```python
from build123d import *

# Parameters (mm, degrees)
BOSS_EXTRUDE1_DEPTH = 20
FILLET2_R           = 2.5
SKETCH2_R           = 2.5
CUT_EXTRUDE1_DEPTH  = 10
SKETCH3_R           = 2.5
CUT_EXTRUDE2_DEPTH  = 10


with BuildPart() as part:
    # Sketch1 → Boss-Extrude1 (new body)
    with BuildSketch(Plane.XY):
        Polygon((0, 0), (20, 0), (20, 18.325792173), (42, 18.325792173), (42, 1.536318489), (62, 1.536318489), (62, 5.536318489), (46, 5.536318489), (46, 22.325792173), (16, 22.325792173), (16, 4), (0, 4), align=None)
    extrude(amount=BOSS_EXTRUDE1_DEPTH)

    # Fillet2
    fillet2_edges = [part.edges().sort_by_distance(p)[0] for p in [
        (16, 4, 10),
        (16, 22.325792173, 10),
        (46, 22.325792173, 10),
        (46, 5.536318489, 10),
    ]]
    fillet(fillet2_edges, radius=FILLET2_R)

    # Sketch2 → Cut-Extrude1 (cut)
    with BuildSketch(Plane(origin=(0, 4, 0), x_dir=(1, 0, 0), z_dir=(0, 1, 0))):
        with Locations((7, -10)):
            Circle(SKETCH2_R)
    extrude(amount=-CUT_EXTRUDE1_DEPTH, mode=Mode.SUBTRACT)

    # Sketch3 → Cut-Extrude2 (cut)
    with BuildSketch(Plane(origin=(0, 5.536318489, 0), x_dir=(1, 0, 0), z_dir=(0, 1, 0))):
        with Locations((55, -10)):
            Circle(SKETCH3_R)
    extrude(amount=-CUT_EXTRUDE2_DEPTH, mode=Mode.SUBTRACT)


solid = part.part
```
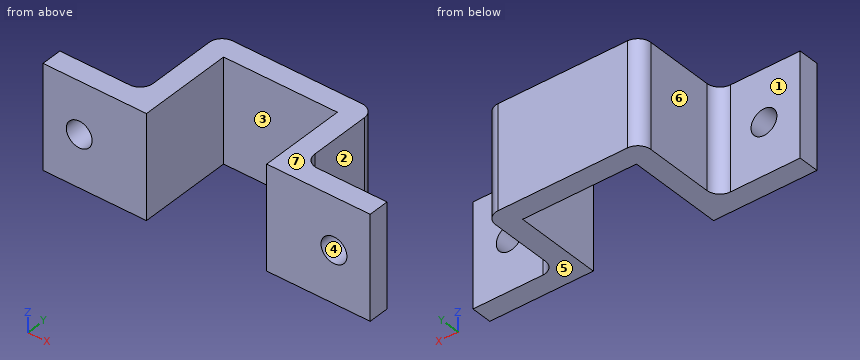
Could you check a few things on this model? Use its own coordinates, in mm. Face numbers are marked on the shaded views. A direction names the side the tool comes from. Coordinates: 2 decimals unless noted, no trailing zeros. Loops run counter-clockwise (first coordinate to the right, second up) from the corner with the lowest first, then second, coordinate; pieces in that order, holes last.
1) Which directions (+Z, -Z, +X, -X, +Y, -Y) give clear straight access to the entire face, cutting with the end or side of a thin tool? Please do the marked faces 1, 2 and 3.
Reported:
face 1: +Z, -Z, -X, +Y
face 2: +Z, -Z, +X, +Y
face 3: +Z, -Z, -Y
2) Imagine slicing it at A-A (y = 2.5). List the corners of the cut face in (x, z) for me, and give its area (3 significant figures).
Reported:
outline: (0, 0) - (20, 0) - (20, 20) - (0, 20) - close; (42, 0) - (62, 0) - (62, 20) - (42, 20) - close; hole circle Ø5 at (7, 10); hole circle Ø5 at (55, 10)
area: 761 mm2
3) Will these pins go through, and if not, where does the flat tip stop? pin 1 Ø12 at (x, z) = (49, 13.5) entering from -Y; pin 2 Ø8 at (x, z) = (7, 10) entering from +Y; pin 3 Ø1.5 at (y, z) = (15, 13) entering from +X.
Reported:
pin 1: stops at y = 1.54
pin 2: stops at y = 4
pin 3: stops at x = 46
4) Please list where these lines run through material, in increasing order: line 1 along X through (y, z) = (3.45, 10); line 2 along X through (y, z) = (17.75, 12.25); line 3 along Z through (x, y) = (7, 0.95).
Reported:
line 1: x = 0 to 4.5, 9.5 to 20, 42 to 52.5, 57.5 to 62
line 2: x = 16 to 20, 42 to 46
line 3: z = 0 to 7.5, 12.5 to 20
5) Thinking about a two-plate mould opening in Z: for the marked faces 4, 5, 6 and 7, which applies, released by +Z, released by -Z, zero draft, split by the parting line, or undercut?
Reported:
face 4: undercut
face 5: released by -Z
face 6: zero draft
face 7: released by +Z
6) Imagine slicing it at B-B (x = 55). List the corners of the cut face in (y, z) for me.
Reported:
outline: (1.54, 0) - (5.54, 0) - (5.54, 7.5) - (1.54, 7.5) - close; (1.54, 12.5) - (5.54, 12.5) - (5.54, 20) - (1.54, 20) - close
7) Imagine slicing it at C-C (z = 10). List the corners of the cut face in (x, y) for me.
Reported:
outline: (0, 0) - (4.5, 0) - (4.5, 4) - (0, 4) - close; (9.5, 0) - (20, 0) - (20, 18.33) - (42, 18.33) - (42, 1.54) - (52.5, 1.54) - (52.5, 5.54) - (48.5, 5.54) arc R2.5 cw to (46, 8.04) - (46, 19.83) arc R2.5 ccw to (43.5, 22.33) - (18.5, 22.33) arc R2.5 ccw to (16, 19.83) - (16, 6.5) arc R2.5 cw to (13.5, 4) - (9.5, 4) - close; (57.5, 1.54) - (62, 1.54) - (62, 5.54) - (57.5, 5.54) - close
8) Imagine slicing it at D-D (y = 9.5). List the corners of the cut face in (x, z) for me, and give its area (3 significant figures).
Reported:
outline: (16, 0) - (20, 0) - (20, 20) - (16, 20) - close; (42, 0) - (46, 0) - (46, 20) - (42, 20) - close
area: 160 mm2
